```python
from build123d import *

# Parameters (mm, degrees)
SKETCH1_W           = 90
SKETCH1_H           = 70
BOSS_EXTRUDE1_DEPTH = 5
SKETCH2_W           = 90
SKETCH2_H           = 70
SKETCH2_W_2         = 80
SKETCH2_H_2         = 60
BOSS_EXTRUDE2_DEPTH = 80
SKETCH3_W           = 70
SKETCH3_H           = 3
BOSS_EXTRUDE4_DEPTH = 6.25
SKETCH4_W           = 4
SKETCH4_H           = 70
BOSS_EXTRUDE5_DEPTH = 40
SKETCH5_W           = 70
SKETCH5_H           = 60
CUT_EXTRUDE3_DEPTH  = 85
FILLET1_R           = 10
FILLET2_R           = 2
FILLET3_R           = 2
FILLET4_R           = 10


with BuildPart() as part:
    # Sketch1 → Boss-Extrude1 (new body)
    with BuildSketch(Plane(origin=(0, 0, 0), x_dir=(1, 0, 0), z_dir=(0, 1, 0))):
        with Locations((45, -35)):
            Rectangle(SKETCH1_W, SKETCH1_H)
    extrude(amount=BOSS_EXTRUDE1_DEPTH)

    # Sketch2 → Boss-Extrude2 (add)
    with BuildSketch(Plane(origin=(0, 5, 0), x_dir=(1, 0, 0), z_dir=(0, 1, 0))):
        with Locations((45, -35)):
            Rectangle(SKETCH2_W, SKETCH2_H)
        with Locations((45, -35)):
            Rectangle(SKETCH2_W_2, SKETCH2_H_2, mode=Mode.SUBTRACT)
    extrude(amount=BOSS_EXTRUDE2_DEPTH)

    # Sketch3 → Boss-Extrude4 (add)
    with BuildSketch(Plane.ZY):
        with Locations((35, 83.5)):
            Rectangle(SKETCH3_W, SKETCH3_H)
    extrude(amount=BOSS_EXTRUDE4_DEPTH)

    # Sketch4 → Boss-Extrude5 (add)
    with BuildSketch(Plane.XZ.offset(-82)):
        with Locations((-4.25, 35)):
            Rectangle(SKETCH4_W, SKETCH4_H)
    extrude(amount=BOSS_EXTRUDE5_DEPTH)

    # Sketch5 → Cut-Extrude3 (cut)
    with BuildSketch(Plane(origin=(90, 0, 0), x_dir=(0, 0, -1), z_dir=(1, 0, 0))):
        with Locations((-35, 55)):
            Rectangle(SKETCH5_W, SKETCH5_H)
    extrude(amount=-CUT_EXTRUDE3_DEPTH, mode=Mode.SUBTRACT)

    # Fillet1
    fillet1_edges = [part.edges().sort_by_distance(p)[0] for p in [
        (5, 5, 35),
        (45, 5, 65),
        (85, 5, 35),
        (45, 5, 5),
    ]]
    fillet(fillet1_edges, radius=FILLET1_R)

    # Fillet2
    # the kernel refuses this fillet: 2 mm, written as the material it adds along each edge
    with BuildSketch(Plane(origin=(0, 82, 70), x_dir=(-1, 0, 0), z_dir=(0, 0, -1)), Plane(origin=(-2.25, 82, 70), x_dir=(0, -1, 0), z_dir=(0, 0, -1))) as fillet2_piece_1:
        with BuildLine():
            CenterArc((FILLET2_R, -FILLET2_R), FILLET2_R, 90, 90)
            Line((0, -FILLET2_R), (0, 0))
            Line((0, 0), (FILLET2_R, 0))
        make_face()
    extrude(amount=70)

    # Fillet3
    fillet3_edges = [part.edges().sort_by_distance(p)[0] for p in [
        (45, 25, 5),
        (85, 25, 35),
        (45, 25, 65),
    ]]
    fillet(fillet3_edges, radius=FILLET3_R)

    # Fillet4
    fillet4_edges = [part.edges().sort_by_distance(p)[0] for p in [
        (90, 12.5, 0),
        (90, 12.5, 70),
    ]]
    fillet(fillet4_edges, radius=FILLET4_R)


solid = part.part
```
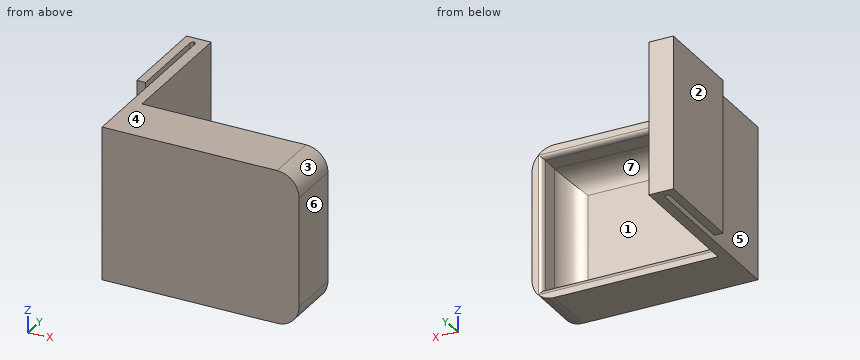
Verification items for the finished model (mm, model axes). Face numbers are marked on the shaded views. A direction names the side the tool comes from. Give positions to 0.01 mm unless a question says otherwise; leave off trailing zeros. Order: outer loops, then holes, each group sorted by start corner. A loop starts at its lowest first (then second) coordinate and runs counter-clockwise, first axis right, second up. Notation, with made-up numbers: M 44,13 L 87,13 A33 ccw 87,48 Z; hole C 82,-31.5 d2. An arc over 180 degrees is marked long. Return JSON: item names as keys, results as strings. Group by question number.
1) Mould release check, pull along X, two halves, no side actions. Record for the marked faces 1, 2, 3 and 4: pulls with the +X half, pulls with the -X half, needs draft (parallel to the pull), parting line crosses it, or undercut.
2) Section check B-B on x = 52.5. Record the cut outline in (y, z).
3) Section check D-D on y = 12.5. Record the cut outline in (x, z), and give its area (3 significant figures).
4) Scan lines: line 1 (X direction, y = 48.5, z = 12); line 2 (X direction, y = 27, z = 58); line 3 (Z direction, x = 42, y = 17.5). Record each from-to range of solid material in increasing order.
5) Section check C-C on z = 27. Record the cut outline in (x, y) (3 decimals).
6) Section check A-A on y = 50.5. Record the cut outline in (x, z), and give its area (3 significant figures).
7) Access from +Z, -Z, +X, -X, +Y, -Y to the whole of each face (thin tool, end or side, straight path). Record for the marked faces 5, 6 and 7.
8) Go/stop test with flat-tipped pins: pin 1 Ø9 at (y, z) = (17.5, 22.5) entering from -X; pin 2 Ø12 at (x, z) = (51.5, 39.5) entering from +Y; pin 3 Ø5 at (y, z) = (46, 18) entering from +X. Record where each tip stops, or that it passes through.
Answer block:
{
 "1": {"face 1": "undercut", "face 2": "pulls with the -X half", "face 3": "pulls with the +X half", "face 4": "needs draft"},
 "2": {"outline": "M 0,0 L 25,0 L 25,3 A2 ccw 23,5 L 15,5 A10 cw 5,15 L 5,55 A10 cw 15,65 L 23,65 A2 ccw 25,67 L 25,70 L 0,70 Z"},
 "3": {"outline": "M 0,0 L 80,0 A10 ccw 90,10 L 90,60 A10 ccw 80,70 L 0,70 Z; hole M 5.32,5.32 L 84.68,5.32 L 84.68,64.68 L 5.32,64.68 Z", "area": "1,550 mm^2"},
 "4": {"line 1": "x = -6.25 to -2.25, 0 to 5", "line 2": "x = 0 to 5", "line 3": "z = 0 to 5, 65 to 70"},
 "5": {"outline": "M -6.25,42 L -2.25,42 L -2.25,80 A2 cw -1.125,81.798 A2 cw 0,80 L 0,0 L 90,0 L 90,25 L 87,25 A2 ccw 85,23 L 85,15 A10 cw 75,5 L 15,5 A10 cw 5,15 L 5,85 L -6.25,85 Z"},
 "6": {"outline": "M -6.25,0 L -2.25,0 L -2.25,70 L -6.25,70 Z; M 0,0 L 5,0 L 5,70 L 0,70 Z", "area": "630 mm^2"},
 "7": {"face 5": "+Z, -Z, -Y", "face 6": "+Z, -Z, +X, +Y, -Y", "face 7": "+Y"},
 "8": {"pin 1": "stops at x = 0", "pin 2": "stops at y = 5", "pin 3": "stops at x = 5"}
}
